```python
from build123d import *

# Parameters (mm, degrees)
BOSS_EXTRUDE1_DEPTH                             = 2
CSK_FOR_M2_FLAT_HEAD_MACHINE_SCREW1_D           = 2.2
CSK_FOR_M2_FLAT_HEAD_MACHINE_SCREW1_DEPTH       = 4
CSK_FOR_M2_FLAT_HEAD_MACHINE_SCREW1_CSINK_D     = 4.4
CSK_FOR_M2_FLAT_HEAD_MACHINE_SCREW1_CSINK_ANGLE = 90
CSK_FOR_M2_FLAT_HEAD_MACHINE_SCREW1_TIP         = 0.660946681
SKETCH9_W                                       = 14
SKETCH9_H                                       = 15
CUT_EXTRUDE4_DEPTH                              = 1.555
SKETCH10_R                                      = 0.5
CUT_EXTRUDE5_DEPTH                              = 1.555
CSK_FOR_M2_FLAT_HEAD_MACHINE_SCREW2_D           = 2.4
CSK_FOR_M2_FLAT_HEAD_MACHINE_SCREW2_DEPTH       = 4
CSK_FOR_M2_FLAT_HEAD_MACHINE_SCREW2_CSINK_D     = 4.4
CSK_FOR_M2_FLAT_HEAD_MACHINE_SCREW2_CSINK_ANGLE = 90
CSK_FOR_M2_FLAT_HEAD_MACHINE_SCREW2_TIP         = 0.721032743
SKETCH12_W                                      = 3.3
SKETCH12_H                                      = 5.6
CUT_EXTRUDE6_DEPTH                              = 31.296192101


with BuildPart() as part:
    # Sketch1 → Boss-Extrude1 (new body)
    with BuildSketch(Plane(origin=(0, 0, 0), x_dir=(1, 0, 0), z_dir=(0, 1, 0))):
        Polygon((-10.147286186, 19.79756588), (-10.147286186, -3.30243412), (-6.697286186, -6.30243412), (16.402713814, -6.30243412), (19.852713814, -3.30243412), (19.852713814, 19.79756588), (16.402713814, 22.79756588), (-6.697286186, 22.79756588), align=None)
    extrude(amount=BOSS_EXTRUDE1_DEPTH)

    # CSK for M2 Flat Head Machine Screw1
    with Locations(Plane(origin=(0, 2, 0), x_dir=(1, 0, 0), z_dir=(0, 1, 0))):
        with Locations((-7.347286186, 15.79756588), (17.052713814, 15.79756588), (17.052713814, 0.69756588), (-7.347286186, 0.69756588)):
            CounterSinkHole(CSK_FOR_M2_FLAT_HEAD_MACHINE_SCREW1_D / 2, CSK_FOR_M2_FLAT_HEAD_MACHINE_SCREW1_CSINK_D / 2, depth=CSK_FOR_M2_FLAT_HEAD_MACHINE_SCREW1_DEPTH, counter_sink_angle=CSK_FOR_M2_FLAT_HEAD_MACHINE_SCREW1_CSINK_ANGLE)
            with Locations((0, 0, -(CSK_FOR_M2_FLAT_HEAD_MACHINE_SCREW1_DEPTH + CSK_FOR_M2_FLAT_HEAD_MACHINE_SCREW1_TIP / 2))):  # 118° drill point
                Cone(0, CSK_FOR_M2_FLAT_HEAD_MACHINE_SCREW1_D / 2, CSK_FOR_M2_FLAT_HEAD_MACHINE_SCREW1_TIP, mode=Mode.SUBTRACT)

    # Sketch9 → Cut-Extrude4 (cut)
    with BuildSketch(Plane(origin=(0, 0, 0), x_dir=(1, 0, 0), z_dir=(0, 1, 0))):
        with Locations((4.852713814, 8.24756588)):
            Rectangle(SKETCH9_W, SKETCH9_H)
    extrude(amount=CUT_EXTRUDE4_DEPTH, mode=Mode.SUBTRACT)

    # Sketch10 → Cut-Extrude5 (cut)
    with BuildSketch(Plane.XZ.offset(-1.555)):
        with Locations(Location((0.352713814, -3.24756588, 0), (0, 0, 270))):
            Circle(SKETCH10_R)
        with Locations(Location((9.352713814, -3.24756588, 0), (0, 0, 270))):
            Circle(SKETCH10_R)
    extrude(amount=-CUT_EXTRUDE5_DEPTH, mode=Mode.SUBTRACT)

    # CSK for M2 Flat Head Machine Screw2
    with Locations(Plane(origin=(9.352713814, 2, -3.24756588), x_dir=(0, 0, 1), z_dir=(0, 1, 0))):
        with Locations((0, 0), (0, -9)):
            CounterSinkHole(CSK_FOR_M2_FLAT_HEAD_MACHINE_SCREW2_D / 2, CSK_FOR_M2_FLAT_HEAD_MACHINE_SCREW2_CSINK_D / 2, depth=CSK_FOR_M2_FLAT_HEAD_MACHINE_SCREW2_DEPTH, counter_sink_angle=CSK_FOR_M2_FLAT_HEAD_MACHINE_SCREW2_CSINK_ANGLE)
            with Locations((0, 0, -(CSK_FOR_M2_FLAT_HEAD_MACHINE_SCREW2_DEPTH + CSK_FOR_M2_FLAT_HEAD_MACHINE_SCREW2_TIP / 2))):  # 118° drill point
                Cone(0, CSK_FOR_M2_FLAT_HEAD_MACHINE_SCREW2_D / 2, CSK_FOR_M2_FLAT_HEAD_MACHINE_SCREW2_TIP, mode=Mode.SUBTRACT)

    # Sketch12 → Cut-Extrude6 (cut, through all)
    with BuildSketch(Plane(origin=(0, 2, 0), x_dir=(1, 0, 0), z_dir=(0, 1, 0))):
        with Locations((4.852713814, 4.34756588)):
            Rectangle(SKETCH12_W, SKETCH12_H)
    extrude(amount=-CUT_EXTRUDE6_DEPTH, mode=Mode.SUBTRACT)


solid = part.part
```
Work out the finished part from the listing and answer in its coordinate system (mm). A direction names the side the tool comes from. Round coordinates to 2 decimals unless told otherwise and drop trailing zeros. Loops run counter-clockwise (first coordinate to the right, second up) from the corner with the lowest first, then second, coordinate; pieces in that order, holes last.
(1) The part is cut by section C-C, the plane z = 4.25. Give the vertices of the cut face in (x, y).
Computed values:
outline: (-9.06, 0) - (18.76, 0) - (18.76, 2) - (-9.06, 2) - close
(2) The mould has two halves that part along X. Classify faces 1 (the cylindrical face through (-8.363, 0.444, -0.276)), 2 (the flat face through (-10.147, 1, -8)), 3 (the flat face through (5, 0, 1)), 4 (the flat face through (18.104, 0.986, 4.823)): pulls with the +X half, pulls with the -X half, needs draft (parallel to the pull), parting line crosses it, or undercut.
Computed values:
face 1: undercut
face 2: pulls with the -X half
face 3: needs draft
face 4: pulls with the +X half
(3) Each of these flat-tipped pins is pushed along its axis until it touches: P1, Ø1.8, axis at x = -7.35, z = -15.8, coming from the +Y side; P2, Ø1, axis at x = 9.5, z = -9, coming from the -Y side (3 decimals). Where does it stop, or does it pass through?
Computed values:
P1: passes through
P2: stops at y = 1.555
(4) Find the intervals of material crossed by L1, parallel to X at y = 1.4, z = -5.5; L2, parallel to Z at x = 7.75, y = 0.9; L3, parallel to Z at x = -7.75, y = 0.7, in increasing order.
Computed values:
L1: x = -10.15 to -2.15, 11.85 to 19.85
L2: z = -22.8 to -15.75, -0.75 to 6.3
L3: z = -21.88 to -16.82, -14.77 to -1.72, 0.33 to 5.39
(5) The part is cut by section A-A, the plane z = -9. Give the vertices of the cut face in (x, y) (3 decimals), and give its area (3 significant figures).
Computed values:
outline: (-10.147, 0) - (-2.147, 0) - (-2.147, 1.555) - (11.853, 1.555) - (11.853, 0) - (19.853, 0) - (19.853, 2) - (-10.147, 2) - close
area: 38.2 mm2
(6) The part is cut by section B-B, the plane y = 0.3. Give the vertices of the cut face in (x, z).
Computed values:
outline: (-10.15, -19.8) - (-6.7, -22.8) - (16.4, -22.8) - (19.85, -19.8) - (19.85, 3.3) - (16.4, 6.3) - (-6.7, 6.3) - (-10.15, 3.3) - close; hole circle Ø2.2 at (-7.35, -15.8); hole circle Ø2.2 at (-7.35, -0.7); hole (-2.15, -15.75) - (11.85, -15.75) - (11.85, -0.75) - (-2.15, -0.75) - close; hole circle Ø2.2 at (17.05, -15.8); hole circle Ø2.2 at (17.05, -0.7)
(7) For faces 5 (the flat face through (18.15, 0.99, -21.28)), 6 (the flat face through (-2.147, 1, -8)), determine the directions among +Z, -Z, +X, -X, +Y, -Y from which every point of the face is accessible in a straight line to the end or side of a thin tool.
Computed values:
face 5: -Z, +X, +Y, -Y
face 6: -Y
